Geometry check sheet. Reference: drawing and pictorial views, mm from the part's lowest x, y, z. Give positions to 0.01 mm unless a question says otherwise; leave off trailing zeros. Write each loop counter-clockwise with the first axis right and the second up, starting at its lowest first coordinate (ties: lowest second). Pieces come first, ordered by that corner, then holes. Notation, with made-up numbers: M 49.25,20 L 56.25,20 A10 ccw 56.25,29 Z; hole C 87,76 d11. An arc over 180 degrees is marked long. Write item = value, one per line. Start each with the question number.
1) Cross-section at A-A, the plane y = 0.3. Record the cut outline in (x, z) (1 decimal), plus the area to 3 significant figures.
2) Cross-section at B-B, the plane x = 31. Record the cut outline in (y, z), plus the area to 3 significant figures.
3) Cross-section at C-C, the plane z = 28.5. Record the cut outline in (x, y).
4) Scan lines: line 1 along Z through (x, y) = (36.5, 0.8); line 2 along Z through (x, y) = (50, 0.5); line 3 along X through (y, z) = (0.6, 8). Record each from-to range of solid material in increasing order. Write a range as [from, to].
5) Go/stop test with a flat-tipped pin: pin 1 (6 mm diameter, centred on x = 53.5, z = 37, fed in from -Y). Record where the tip stops, or that it passes through.
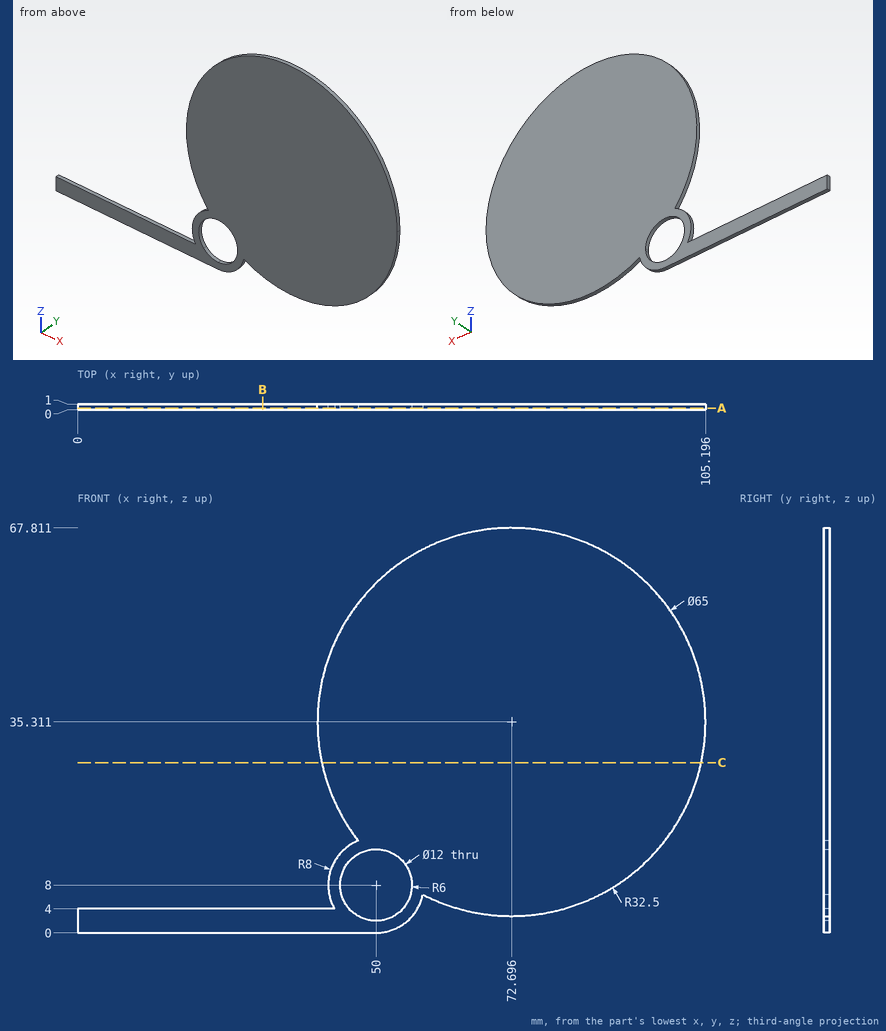
Reply:
q1.outline = M 0,0 L 50,0 A8 ccw 57.8,6.4 A32.5 ccw long 47,15.4 A8 ccw 43.1,4 L 0,4 Z; hole C 50,8 d12
q1.area = 3,540 mm2
q2.outline = M 0,0 L 1,0 L 1,4 L 0,4 Z
q2.area = 4.00 mm2
q3.outline = M 40.92,0 L 104.47,0 L 104.47,1 L 40.92,1 Z
q4.line_1 = [0, 4]
q4.line_2 = [0, 2], [14, 58.57]
q4.line_3 = [42, 44], [56, 90.31]
q5.pin_1 = 0
